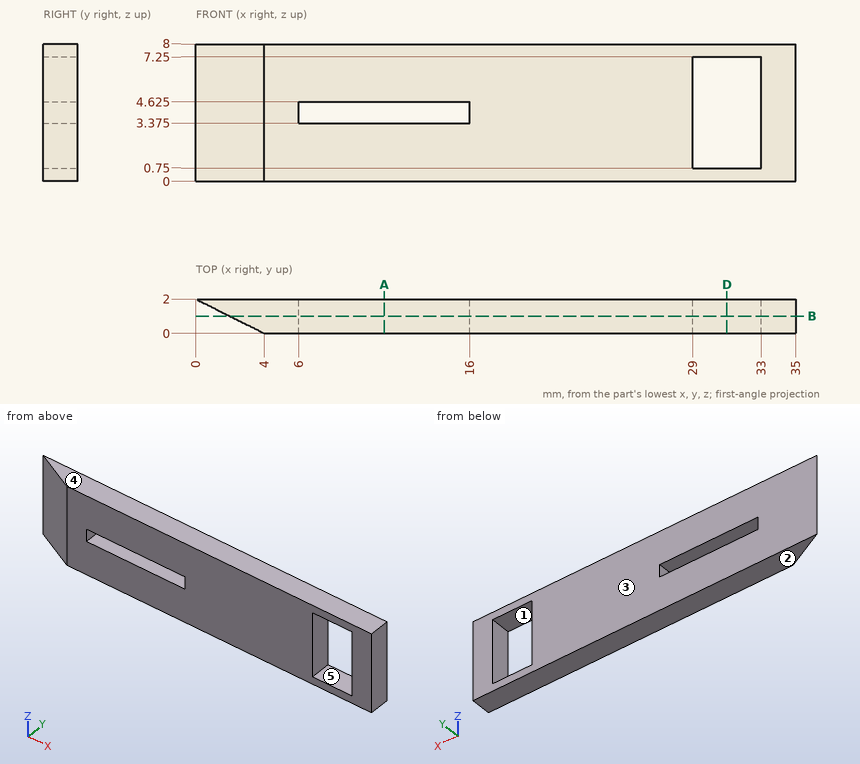
The figure shows three views and two pictorial views of one solid part (mm, origin at its lowest corner). Answer the questions. A direction names the side the tool comes from. Round coordinates to 2 decimals unless told otherwise and drop trailing zeros. Write each loop counter-clockwise with the first axis right and the second up, starting at its lowest first coordinate (ties: lowest second). Pieces come first, ordered by that corner, then holes. Notation, with made-up numbers: M 51,29 L 59,29 A22 cw 59,54 Z; hole C 68.25,75 d4. An arc over 180 degrees is marked long. Write each question's results on one line, items separated by ' | '. Start each with the question number.
(1) Determine the mould class of the marked faces 3, 4 and 5 for opening direction Z: +Z half, -Z half, draft (parallel to the pull), parting line (faces both ways), or undercut.
(2) The part is cut by section A-A, the plane x = 11. Write down the section's boundary in (y, z) (3 decimals), and give its area (3 significant figures).
(3) The part is cut by section D-D, the plane x = 31. Write down the section's boundary in (y, z).
(4) This flat-tipped pin is pushed along its axis until it touches: P1, Ø0.6, axis at y = 1.5, z = 3.5, coming from the -X side. Where does it stop, or does it pass through?
(5) For the marked faces 1 and 2, determine the directions among +Z, -Z, +X, -X, +Y, -Y from which every point of the face is accessible in a straight line to the end or side of a thin tool.
(6) The part is cut by section B-B, the plane y = 1. Write down the section's boundary in (x, z) (3 decimals).
(7) Find the intervals of material crossed by line 1 (Z direction, x = 11, y = 1.95) (3 decimals); line 2 (X direction, y = 0.9, z = 4.5); line 3 (Z direction, x = 31.5, y = 1.1), in increasing order.
Worked answers:
1) face 3: draft | face 4: +Z half | face 5: undercut
2) outline: M 0,0 L 2,0 L 2,3.375 L 0,3.375 Z; M 0,4.625 L 2,4.625 L 2,8 L 0,8 Z | area: 13.5 mm²
3) outline: M 0,0 L 2,0 L 2,0.75 L 0,0.75 Z; M 0,7.25 L 2,7.25 L 2,8 L 0,8 Z
4) P1: stops at x = 0.4
5) face 1: +Y, -Y | face 2: -Z, +X, -X, +Y, -Y
6) outline: M 2,0 L 35,0 L 35,8 L 2,8 Z; hole M 6,3.375 L 16,3.375 L 16,4.625 L 6,4.625 Z; hole M 29,0.75 L 33,0.75 L 33,7.25 L 29,7.25 Z
7) line 1: z = 0 to 3.375, 4.625 to 8 | line 2: x = 2.2 to 6, 16 to 29, 33 to 35 | line 3: z = 0 to 0.75, 7.25 to 8
